from build123d import *

# Parameters (mm, degrees)
CHAMBRAGE_POUR_VIS_T_TE_HEXAGONALE_M41_D           = 4.5
CHAMBRAGE_POUR_VIS_T_TE_HEXAGONALE_M41_CBORE_D     = 8
CHAMBRAGE_POUR_VIS_T_TE_HEXAGONALE_M41_CBORE_DEPTH = 5
R_P_TITION_CIRCULAIRE1_COUNT                       = 3


with BuildPart() as part:
    # Esquisse1 → Révolution1 (revolve)
    with BuildSketch(Plane.XY, mode=Mode.PRIVATE) as r_volution1_sk:
        Polygon((0, 20), (0, 33), (7, 33), (7, 23.5), (4, 23.5), (4, 20), align=None)
    revolve(r_volution1_sk.sketch.rotate(Axis((-15.138230384, 0, 0), (1, 0, 0)), 90), axis=Axis((-15.138230384, 0, 0), (1, 0, 0)))

    # Chambrage pour vis à tête hexagonale M41 (through all)
    with Locations(Plane(origin=(0, 27.984819093, -0.921900388), x_dir=(0, 0, -1), z_dir=(-1, 0, 0))):
        with Locations((0, 0)):
            chambrage_pour_vis_t_te_hexagonale_m41 = CounterBoreHole(CHAMBRAGE_POUR_VIS_T_TE_HEXAGONALE_M41_D / 2, CHAMBRAGE_POUR_VIS_T_TE_HEXAGONALE_M41_CBORE_D / 2, CHAMBRAGE_POUR_VIS_T_TE_HEXAGONALE_M41_CBORE_DEPTH)

    # Répétition circulaire1: Chambrage pour vis à tête hexagonale M41 ×3 about axis
    r_p_tition_circulaire1_axis = Axis((0, 0, 0), (1, 0, 0))
    for i in range(1, R_P_TITION_CIRCULAIRE1_COUNT):
        add(chambrage_pour_vis_t_te_hexagonale_m41.rotate(r_p_tition_circulaire1_axis, i * 360 / R_P_TITION_CIRCULAIRE1_COUNT), mode=Mode.SUBTRACT)


solid = part.part
Can you work these out from the model? Positions are in its coordinate system, mm. A direction names the side the tool comes from. Round coordinates to 2 decimals unless told otherwise and drop trailing zeros. Loops run counter-clockwise (first coordinate to the right, second up) from the corner with the lowest first, then second, coordinate; pieces in that order, holes last. Notation, with made-up numbers: (36.25, 57) - (71.25, 57) arc R31 ccw to (71.25, 83) - close; hole circle Ø11 at (37, 43.5). An arc over 180 degrees is marked (long way). Write item = value, one per line. Start each with the question number.
(1) If we section it at A-A (y = 0): Please give me the cut outline in (x, z).
(2) For faces 4 (the face through (6.014, -15.425, 24.404)), 5 (the face through (4, -19, 7)), 6 (the face through (5, 30, -3)), which set-ups out of +Z, -Z, +X, -X, +Y, -Y let a thin tool reach every point of the face, with its end or its side?
(3) If we section it at B-B (z = -15): Please give me the cut outline in (x, y), and give its area (3 significant figures).
(4) If I drill on probe 1 along Y at (x, z) = (4.75, -4); probe 2 along Y at (x, z) = (1.3, 0); probe 3 along Z at (x, y) = (4.5, -12.5), over which ranges is the centre line in solid material (lowest first)? Write a range as [from, to].
(5) If we section it at D-D (z = 0): Please give me the cut outline in (x, y), and give its area (3 significant figures).
(6) For P1, Ø7, axis at y = -14.79, z = -23.77, coming from the -X side; P2, Ø10.5, axis at y = 27.98, z = -0.92, coming from the +X side; P3, Ø2, axis at x = 4.5, y = -20.5, coming from the +Z side; P4, Ø2.5, axis at y = 27.5, z = -1, coming from the -X side, each with a flat end and sliding along its axis, tell me the tip position at first contact or that it passes through.
(7) If we section it at C-C (x = 1.5): Please give me the cut outline in (y, z), and give its area (3 significant figures).
(8) If we mould it in two halves opening along Z, with no side actions, what happens to faces 1 (the face through (3.549, -9.912, 31.476)), 2 (the face through (0, 22, 0)), 3 (the face through (1.97, -0.88, -19.98))? For each: released by +Z, released by -Z, zero draft, split by the parting line, or undercut.
Ans:
q1.outline = (0, -33) - (7, -33) - (7, -23.5) - (4, -23.5) - (4, -20) - (0, -20) - close; (0, 20) - (4, 20) - (4, 23.5) - (7, 23.5) - (7, 33) - (0, 33) - close
q2.face_4 = +X, -X
q2.face_5 = +X
q2.face_6 = -X
q3.outline = (0, -29.39) - (7, -29.39) - (7, -18.09) - (4, -18.09) - (4, -13.23) - (0, -13.23) - close; (0, 13.23) - (4, 13.23) - (4, 18.09) - (7, 18.09) - (7, 29.39) - (0, 29.39) - close
q3.area = 197 mm²
q4.probe_1 = [-32.76, -23.16], [23.16, 25.43], [30.54, 32.76]
q4.probe_2 = [-33, -20], [20, 24.09], [31.88, 33]
q4.probe_3 = [-30.54, -27.05], [-20.5, -19.9], [19.9, 20.76], [28.64, 30.54]
q5.outline = (0, -33) - (7, -33) - (7, -23.5) - (4, -23.5) - (4, -20) - (0, -20) - close; (0, 20) - (4, 20) - (4, 23.5) - (7, 23.5) - (7, 25.93) - (5, 25.93) - (5, 24.09) - (0, 24.09) - close; (0, 31.88) - (5, 31.88) - (5, 30.04) - (7, 30.04) - (7, 33) - (0, 33) - close
q5.area = 114 mm²
q6.P1 = 5
q6.P2 = 7
q6.P3 = 26.62
q6.P4 = through
q7.outline = circle Ø66 at (0, 0); hole circle Ø40 at (0, 0); hole circle Ø8 at (-14.79, -23.77); hole circle Ø8 at (-13.19, 24.7); hole circle Ø8 at (27.98, -0.92)
q7.area = 2,010 mm²
q8.face_1 = split by the parting line
q8.face_2 = zero draft
q8.face_3 = undercut
